from build123d import *

# Parameters (mm, degrees)
F0_R     = 8
F0_R_2   = 5
F1_DEPTH = 10
F2_DEPTH = 180
F3_SIZE  = 1


with BuildPart() as f1:
    # F0 (on Front) → F1 (new body)
    with BuildSketch(Plane.XZ):
        Circle(F0_R)
        Circle(F0_R_2, mode=Mode.SUBTRACT)
        Circle(F0_R_2)
    extrude(amount=-F1_DEPTH)

    # F0 (on Front) → F2 (join)
    with BuildSketch(Plane.XZ):
        Circle(F0_R_2)
    extrude(amount=F2_DEPTH)

    # F3
    f3_edges = [f1.edges().sort_by_distance(p)[0] for p in [
        (-5, -180, 0),
    ]]
    chamfer(f3_edges, length=F3_SIZE)


solid = f1.part
Geometry: final body of the model. Coordinates: model frame, mm. A direction names the side the tool comes from. Give positions to 0.01 mm unless a question says otherwise; leave off trailing zeros. Write each loop counter-clockwise with the first axis right and the second up, starting at its lowest first coordinate (ties: lowest second). Pieces come first, ordered by that corner, then holes. Notation, with made-up numbers: M 50,9 L 86,9 A21 ccw 86,41 Z; hole C -28.5,46.25 d2. An arc over 180 degrees is marked long. Answer in a Markdown table with one row per item. Add a question column.
(1) First-contact query: pin 1 (6 mm diameter, centred on x = 4, y = -142, fed in from -Z); pin 2 (1.5 mm diameter, centred on x = 0, y = -83, fed in from +Z); pin 3 (5 mm diameter, centred on y = -17.5, z = 0.5, fed in from -X). Flat tips, straight axial feed; report the tip coordinate or a pass-through.
(2) Section B-B on z = 0. Return loops of the section in (x, y).
(3) Ray query, line 1 (Z direction, x = -3, y = -167); line 2 (Y direction, x = -1.5, z = -6.75); line 3 (Z direction, x = 0.5, y = -28). Return the intervals inside material, ascending.
(4) Section C-C on y = -120. Return loops of the section in (x, z), and give its area (3 significant figures).
(5) Section A-A on x = 0. Return loops of the section in (y, z).
(6) Reachability of faces 1 (the flat face through (0, 10, 0)), 2 (the flat face through (5.2, 0, 0.1)) from +Z, -Z, +X, -X, +Y, -Y: full face, straight path, thin tool, end or side. Return the list, or none.
Result set:
| question | item | result |
|---|---|---|
| 1 | pin 1 | stops at z = -4.9 |
| 1 | pin 2 | stops at z = 5 |
| 1 | pin 3 | stops at x = -5 |
| 2 | outline | M -8,0 L -5,0 L -5,-179 L -4,-180 L 4,-180 L 5,-179 L 5,0 L 8,0 L 8,10 L -8,10 Z |
| 3 | line 1 | z = -4 to 4 |
| 3 | line 2 | y = 0 to 10 |
| 3 | line 3 | z = -4.97 to 4.97 |
| 4 | outline | C 0,0 d10 |
| 4 | area | 78.5 mm^2 |
| 5 | outline | M -180,-4 L -179,-5 L 0,-5 L 0,-8 L 10,-8 L 10,8 L 0,8 L 0,5 L -179,5 L -180,4 Z |
| 6 | face 1 | +Z, -Z, +X, -X, +Y |
| 6 | face 2 | -Y |
